from build123d import *

# Parameters (mm, degrees)
F0_W     = 118.8637800515
F0_H     = 77.4197466671
F1_DEPTH = 48.768
F4_R     = 30.7965572654
F5_DEPTH = 65.786


# Not quite as in the source:
# - the program builds the solid bodies; features that only make, move or delete a surface that nothing else refers to are left out


with BuildPart() as f1:
    # F0 (on Front) → F1 (new body)
    with BuildSketch(Plane.XZ):
        with Locations((1.8707383424, -0.1439023763)):
            Rectangle(F0_W, F0_H)
    extrude(amount=F1_DEPTH)

    # F4 (on Front) → F5 (join)
    with BuildSketch(Plane.XZ):
        with Locations((0, 46.3367253542)):
            Circle(F4_R)
    extrude(amount=F5_DEPTH)


solid = f1.part
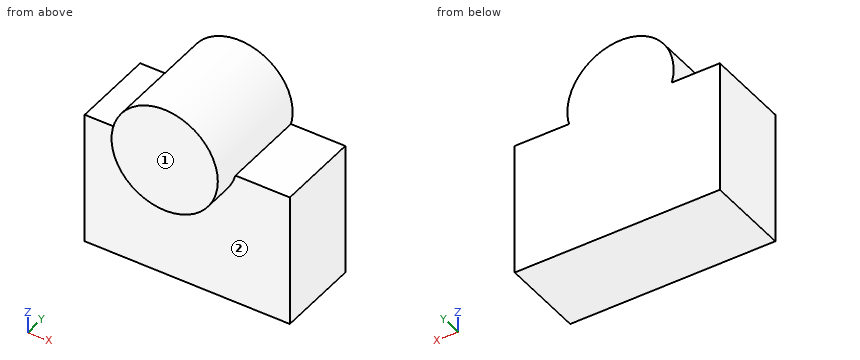
Work out the finished part from the listing and answer in its coordinate system (mm). Face numbers are marked on the shaded views. A direction names the side the tool comes from. Round coordinates to 2 decimals unless told otherwise and drop trailing zeros. Write each loop counter-clockwise with the first axis right and the second up, starting at its lowest first coordinate (ties: lowest second). Pieces come first, ordered by that corner, then holes. Notation, with made-up numbers: M 43.25,24.25 L 63.25,24.25 A20 ccw 63.25,35.25 Z; hole C 18,50.25 d10. An arc over 180 degrees is marked long. Use a Markdown table: item, result.
1) The part is cut by section B-B on x = 0. Give the vertices of the cut face in (y, z).
Taken from the geometry:
| item | result |
|---|---|
| outline | M -65.79,15.54 L -48.77,15.54 L -48.77,-38.85 L 0,-38.85 L 0,77.13 L -65.79,77.13 Z |
2) Flat-ended cylindrical pins translate along their axes: pin 1 (1 mm diameter, centred on y = -24.5, z = 41, fed in from +X); pin 2 (22 mm diameter, centred on x = -38.5, y = -29, fed in from +Z); pin 3 (10 mm diameter, centred on x = -17.5, y = -51, fed in from +Z). Find the tip coordinate at first contact, or state that the pin passes through.
Taken from the geometry:
| item | result |
|---|---|
| pin 1 | stops at x = 30.41 |
| pin 2 | stops at z = 60.2 |
| pin 3 | stops at z = 74.48 |
3) Which of the six approach directions +Z, -Z, +X, -X, +Y, -Y give full straight-line access (tool end or side, diameter ignored) to the marked faces 1 and 2?
Taken from the geometry:
| item | result |
|---|---|
| face 1 | +Z, -Z, +X, -X, -Y |
| face 2 | -Z, -Y |
4) The part is cut by section C-C on z = -17. Give the vertices of the cut face in (x, y).
Taken from the geometry:
| item | result |
|---|---|
| outline | M -57.56,-48.77 L 61.3,-48.77 L 61.3,0 L -57.56,0 Z |
5) The part is cut by section A-A on y = -9.5. Give the vertices of the cut face in (x, z).
Taken from the geometry:
| item | result |
|---|---|
| outline | M -57.56,-38.85 L 61.3,-38.85 L 61.3,38.57 L 29.8,38.57 A30.8 ccw long -29.8,38.57 L -57.56,38.57 Z |
6) Consider line 1 (Y direction, x = -49, z = -22); line 2 (Z direction, x = -37.5, y = -46); line 3 (X direction, y = -14, z = 45). Determine where each line is inside the solid, lowest interval first. Write a range as [from, to].
Taken from the geometry:
| item | result |
|---|---|
| line 1 | y = [-48.77, 0] |
| line 2 | z = [-38.85, 38.57] |
| line 3 | x = [-30.77, 30.77] |
7) The part is cut by section D-D on z = 27.5. Give the vertices of the cut face in (x, y).
Taken from the geometry:
| item | result |
|---|---|
| outline | M -57.56,-48.77 L -24.36,-48.77 L -24.36,-65.79 L 24.36,-65.79 L 24.36,-48.77 L 61.3,-48.77 L 61.3,0 L -57.56,0 Z |
